Source: CAD feature listing. Evaluate the final solid. Frame: model axes, mm. Give positions to 0.01 mm unless a question says otherwise; leave off trailing zeros. Loops run counter-clockwise (first coordinate to the right, second up) from the corner with the lowest first, then second, coordinate; pieces in that order, holes last. Notation, with made-up numbers: M -27,48.25 L 29,48.25 A15 cw 29,61.25 Z; hole C 0.5,69 d1. An arc over 180 degrees is marked long. Write item = value, one per line.
from build123d import *

# Parameters (mm, degrees)
SKETCH_1_R      = 26.5
SKETCH_1_R_2    = 15
SKETCH_1_R_3    = 2.1
EXTRUDE_1_DEPTH = 17


with BuildPart() as part:
    # 草图1 → 凸台-拉伸1 (new body)
    with BuildSketch(Plane.XY):
        Circle(SKETCH_1_R)
        Circle(SKETCH_1_R_2, mode=Mode.SUBTRACT)
        with Locations((0, 21.5)):
            Circle(SKETCH_1_R_3, mode=Mode.SUBTRACT)
        with Locations((16.469955527, 13.819933608)):
            Circle(SKETCH_1_R_3, mode=Mode.SUBTRACT)
        with Locations((21.17336669, -3.73343582)):
            Circle(SKETCH_1_R_3, mode=Mode.SUBTRACT)
        with Locations((0, -21.5)):
            Circle(SKETCH_1_R_3, mode=Mode.SUBTRACT)
        with Locations((-16.469955527, -13.819933608)):
            Circle(SKETCH_1_R_3, mode=Mode.SUBTRACT)
        with Locations((-21.17336669, 3.73343582)):
            Circle(SKETCH_1_R_3, mode=Mode.SUBTRACT)
        with BuildLine():
            ThreePointArc((-8.20848344, 22.552622899), (-15.426902632, 18.385066635), (-20.784609691, 12))
            ThreePointArc((-20.784609691, 12), (-19.869546181, 8.584936491), (-16.454482672, 9.5))
            ThreePointArc((-16.454482672, 9.5), (-12.212964584, 14.554844419), (-6.498382723, 17.854159795))
            ThreePointArc((-6.498382723, 17.854159795), (-5.00420153, 21.058441705), (-8.20848344, 22.552622899))
        make_face(mode=Mode.SUBTRACT)
        with BuildLine():
            ThreePointArc((12, 20.784609691), (10.142838282, 21.751386889), (8.20848344, 22.552622899))
            ThreePointArc((8.20848344, 22.552622899), (5.00420153, 21.058441705), (6.498382723, 17.854159795))
            ThreePointArc((6.498382723, 17.854159795), (8.029746973, 17.219847954), (9.5, 16.454482672))
            ThreePointArc((9.5, 16.454482672), (12.915063509, 17.369546181), (12, 20.784609691))
        make_face(mode=Mode.SUBTRACT)
        with BuildLine():
            ThreePointArc((18.711347307, 3.299315376), (18.352590699, 4.917561857), (17.854159795, 6.498382723))
            ThreePointArc((17.854159795, 6.498382723), (19.348340989, 9.702664633), (22.552622899, 8.20848344))
            ThreePointArc((22.552622899, 8.20848344), (23.182219831, 6.211657082), (23.635386072, 4.167556264))
            ThreePointArc((23.635386072, 4.167556264), (21.607487134, 1.271416437), (18.711347307, 3.299315376))
        make_face(mode=Mode.SUBTRACT)
        with BuildLine():
            ThreePointArc((6.498382723, -17.854159795), (12.212964584, -14.554844419), (16.454482672, -9.5))
            ThreePointArc((16.454482672, -9.5), (19.869546181, -8.584936491), (20.784609691, -12))
            ThreePointArc((20.784609691, -12), (15.426902632, -18.385066635), (8.20848344, -22.552622899))
            ThreePointArc((8.20848344, -22.552622899), (5.00420153, -21.058441705), (6.498382723, -17.854159795))
        make_face(mode=Mode.SUBTRACT)
        with BuildLine():
            ThreePointArc((-9.5, -16.454482672), (-8.029746973, -17.219847954), (-6.498382723, -17.854159795))
            ThreePointArc((-6.498382723, -17.854159795), (-5.00420153, -21.058441705), (-8.20848344, -22.552622899))
            ThreePointArc((-8.20848344, -22.552622899), (-10.142838282, -21.751386889), (-12, -20.784609691))
            ThreePointArc((-12, -20.784609691), (-12.915063509, -17.369546181), (-9.5, -16.454482672))
        make_face(mode=Mode.SUBTRACT)
        with BuildLine():
            ThreePointArc((-23.635386072, -4.167556264), (-23.182219831, -6.211657082), (-22.552622899, -8.20848344))
            ThreePointArc((-22.552622899, -8.20848344), (-19.348340989, -9.702664633), (-17.854159795, -6.498382723))
            ThreePointArc((-17.854159795, -6.498382723), (-18.352590699, -4.917561857), (-18.711347307, -3.299315376))
            ThreePointArc((-18.711347307, -3.299315376), (-21.607487134, -1.271416437), (-23.635386072, -4.167556264))
        make_face(mode=Mode.SUBTRACT)
    extrude(amount=EXTRUDE_1_DEPTH)


solid = part.part
1. Material intervals for probe 1 along Y at (x, z) = (0, 11); probe 2 along X at (y, z) = (6, 1.75); probe 3 along Y at (x, z) = (-7, 16), sorted ascending. Write a range as from..to.
Derived:
probe_1 = -26.5..-23.6, -19.4..-15, 15..19.4, 23.6..26.5
probe_2 = -25.81..-13.75, 13.75..18.03, 23.24..25.81
probe_3 = -25.56..-22.68, -17.66..-13.27, 13.27..17.66, 22.68..25.56
2. Cut plane C-C, the plane z = 15.75. Count the separate pieces of the cut face and the enclosed holes in it, then the cut area to 3 significant figures.
Derived:
separate_pieces = 1
enclosed_holes = 13
area = 1,070 mm²
3. Pull-direction query (X, two-part tool) for faces 1 (the cylindrical face through (14.246, 22.345, 8.381)), 2 (the cylindrical face through (-18.347, -4.94, 8.381)); classes: +X half, -X half, draft (parallel to the pull), parting line (faces both ways), or undercut.
Derived:
face_1 = parting line
face_2 = undercut
4. Cut plane D-D, the plane y = -10.75. Return the cut outline in (x, z).
Derived:
outline = M -24.22,0 L -10.46,0 L -10.46,17 L -24.22,17 Z; M 10.46,0 L 15.67,0 L 15.67,17 L 10.46,17 Z; M 21.12,0 L 24.22,0 L 24.22,17 L 21.12,17 Z
5. Cut plane B-B, the plane x = 0. Return the cut outline in (y, z), then the cut area to 3 significant figures.
Derived:
outline = M -26.5,0 L -23.6,0 L -23.6,17 L -26.5,17 Z; M -19.4,0 L -15,0 L -15,17 L -19.4,17 Z; M 15,0 L 19.4,0 L 19.4,17 L 15,17 Z; M 23.6,0 L 26.5,0 L 26.5,17 L 23.6,17 Z
area = 248 mm²
6. First-contact query: pin 1 Ø10 at (x, y) = (-11, 13.5) entering from -Z; pin 2 Ø6 at (x, z) = (-13, 9) entering from +Y; pin 3 Ø3.5 at (x, y) = (0, 21.5) entering from -Z; pin 4 Ø2 at (y, z) = (19, 8.5) entering from +X. Flat tips, straight axial feed; report the tip coordinate or a pass-through.
Derived:
pin_1 = 0
pin_2 = 24.54
pin_3 = through
pin_4 = 19.45
7. Cut plane A-A, the plane y = 0. Return the cut outline in (x, z), then the cut area to 3 significant figures.
Derived:
outline = M -26.5,0 L -15,0 L -15,17 L -26.5,17 Z; M 15,0 L 26.5,0 L 26.5,17 L 15,17 Z
area = 391 mm²
